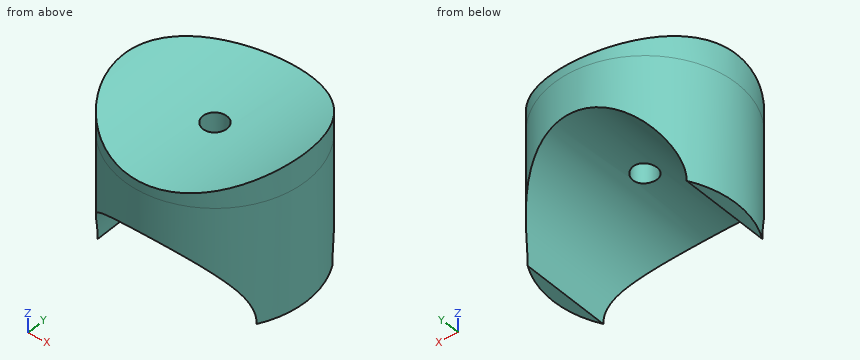
```python
from build123d import *

# Parameters (mm, degrees)
ESBO_O1_R                  = 19
RESSALTO_EXTRUS_O1_DEPTH   = 7.5
CORTE_EXTRUS_O1_DEPTH      = 28.897132469
CORTE_EXTRUS_O1_DEPTH_BACK = 28.897132469
ESBO_O7_R                  = 19
RESSALTO_EXTRUS_O3_DEPTH   = 25
ESBO_O8_R                  = 16.5
CORTE_EXTRUS_O2_DEPTH      = 29
FURO_ROSCADO_DE_M62_D      = 5


with BuildPart() as part:
    # Esboço1 → Ressalto-extrusão1 (new, symmetric)
    with BuildSketch(Plane.XY):
        Circle(ESBO_O1_R)
    extrude(amount=RESSALTO_EXTRUS_O1_DEPTH, both=True)

    # Esboço2 → Corte-extrusão1 (cut, two sides: drawn at the far end of the back side and taken through both)
    with BuildSketch(Plane(origin=(0, 0, 0), x_dir=(1, 0, 0), z_dir=(0, 1, 0)).offset(-CORTE_EXTRUS_O1_DEPTH_BACK)):
        with BuildLine():
            Line((-99.472761542, -34.36341569), (-19, 1.5))
            ThreePointArc((-19, 1.5), (0, 5.542140614), (19, 1.5))
            Line((19, 1.5), (99.472761542, -34.36341569))
            Line((99.472761542, -34.36341569), (99.472761542, -210.568409208))
            Line((99.472761542, -210.568409208), (-99.472761542, -210.568409208))
            Line((-99.472761542, -210.568409208), (-99.472761542, -34.36341569))
        make_face()
    extrude(amount=CORTE_EXTRUS_O1_DEPTH + CORTE_EXTRUS_O1_DEPTH_BACK, mode=Mode.SUBTRACT)

    # Esboço7 → Ressalto-extrusão3 (add)
    with BuildSketch(Plane(origin=(0, 0, -7.5), x_dir=(-1, 0, 0), z_dir=(0, 0, -1))):
        Circle(ESBO_O7_R)
    extrude(amount=RESSALTO_EXTRUS_O3_DEPTH)

    # Esboço8 → Corte-extrusão2 (cut, symmetric)
    with BuildSketch(Plane(origin=(0, 0, 0), x_dir=(1, 0, 0), z_dir=(0, 1, 0))):
        with Locations((0, 32.5)):
            Circle(ESBO_O8_R)
    extrude(amount=CORTE_EXTRUS_O2_DEPTH, both=True, mode=Mode.SUBTRACT)

    # Furo roscado de M62 (through all)
    with Locations(Plane.XY):
        with Locations((0, 0)):
            Hole(FURO_ROSCADO_DE_M62_D / 2)


solid = part.part
```
The listing builds one solid part. Answer for the finished solid, in the listing's coordinates (mm). Round coordinates to 2 decimals unless told otherwise and drop trailing zeros. Loops run counter-clockwise (first coordinate to the right, second up) from the corner with the lowest first, then second, coordinate; pieces in that order, holes last. Notation, with made-up numbers: (67, -8) - (121, -8) arc R22 ccw to (121, 21) - close; hole circle Ø7 at (24, 86.25). An arc over 180 degrees is marked (long way). Use one line per item in the form item = value. Start each with the question number.
1. Consider line 1 (Y direction, x = 0, z = -11.5); line 2 (X direction, y = -3.5, z = -31). Determine where each line is inside the solid, lowest interval first. Write a range as [from, to].
2. The part is cut by section A-A on x = 0. Determine the outline of the cut face in (y, z), then the cut area to 3 significant figures.
3. The part is cut by section B-B on y = 0. Determine the outline of the cut face in (x, z).
4. Given pin 1 Ø1 at (y, z) = (-15, -20.5) entering from -X; pin 2 Ø6 at (x, y) = (0, 0) entering from +Z; pin 3 Ø1.5 at (x, z) = (-15, -9.5) entering from -Y, each flat-ended and moving along its own axis, determine where each tip first touches the part or whether it passes through.
5. The part is cut by section C-C on z = -10. Determine the outline of the cut face in (x, y), then the cut area to 3 significant figures.
6. The part is cut by section D-D on y = -4. Determine the outline of the cut face in (x, z), then the cut area to 3 significant figures.
Geometry check:
q1.line_1 = [-19, -2.5], [2.5, 19]
q1.line_2 = [-18.67, -16.43], [16.43, 18.67]
q2.outline = (-19, -16) - (-2.5, -16) - (-2.5, -5.54) - (-19, -5.54) - close; (2.5, -16) - (19, -16) - (19, -5.54) - (2.5, -5.54) - close
q2.area = 345 mm^2
q3.outline = (-19, -32.5) - (-16.5, -32.5) arc R16.5 cw to (-2.5, -16.19) - (-2.5, -5.48) arc R46.68 cw to (-19, -1.5) - close; (2.5, -16.19) arc R16.5 cw to (16.5, -32.5) - (19, -32.5) - (19, -1.5) arc R46.68 cw to (2.5, -5.48) - close
q4.pin_1 = -12.28
q4.pin_2 = -5.45
q4.pin_3 = -12.57
q5.outline = circle Ø38 at (0, 0); hole circle Ø5 at (0, 0)
q5.area = 1,110 mm^2
q6.outline = (-18.57, -32.5) - (-16.5, -32.5) arc R16.5 cw to (16.5, -32.5) - (18.57, -32.5) - (18.57, -1.69) arc R46.68 cw to (-18.57, -1.69) - close
q6.area = 621 mm^2
